Geometry: final body of the model. Coordinates: model frame, mm. A direction names the side the tool comes from. Give positions to 0.01 mm unless a question says otherwise; leave off trailing zeros. Loops run counter-clockwise (first coordinate to the right, second up) from the corner with the lowest first, then second, coordinate; pieces in that order, holes last. Notation, with made-up numbers: (63, 13) -> (119, 13) arc R14 ccw to (119, 32) -> close; hole circle Ø2 at (3.25, 59.25). An arc over 180 degrees is marked (long way). Answer in a Markdown table with one row per item. Add a question column.
1) First-contact query: P1, Ø3, axis at x = 21.5, y = 46, coming from the -Z side; P2, Ø10, axis at x = 134.5, z = -18, coming from the +Y side; P3, Ø10, axis at x = 39, y = -173, coming from the +Z side. Flat tips, straight axial feed; report the tip coordinate or a pass-through.
2) Section query A-A (x = -71). Return the cut outline in (y, z).
3) Line query: line 1 (Y direction, x = -7.5, z = 64); line 2 (X direction, y = -11.5, z = 64.5); line 3 (Y direction, x = 137, z = 19). Output: solid intervals per line, ascending. Write a range as from..to.
4) Draft query along Y for faces 1 (the flat face through (38, -292.151, 36)), 2 (the flat face through (39, -157.151, 35)), 3 (the flat face through (13, -150, 70)), 4 (the flat face through (31, 202.849, 35)). Return one class per face: +Y half, -Y half, draft (parallel to the pull), parting line (faces both ways), or undercut.
5) Section query D-D (x = -150). Return the cut outline in (y, z), plus the area to 3 significant figures.
6) Access query for faces 5 (the flat face through (0, -216, 13)), 6 (the flat face through (80, -216, 12)), 7 (the flat face through (32, 25, 60)), 8 (the flat face through (31, 20, 0)). Directions: +Z, -Z, +X, -X, +Y, -Y. A direction counts if a zero-diameter tool reaches every point of the face in a straight line with its end or side. Return the directions, or none.
7) Section query B-B (y = 135). Return the cut outline in (x, z), plus the area to 3 significant figures.
8) Section query C-C (z = 82). Return the cut outline in (x, y).
Autodesk Inventor part; units mm, degrees
ref_plane "YZ Plane" through (0, 0, 0) normal (1, 0, 0) x (0, 1, 0)
ref_plane "XZ Plane" through (0, 0, 0) normal (0, 1, 0) x (-1, 0, 0)
ref_plane "XY Plane" through (0, 0, 0) normal (0, 0, 1) x (1, 0, 0)
sketch "Esquisse1" plane through (0, 0, 0) normal (0, 0, 1) x (1, 0, 0)
  line L0 (-242.3239, 202.8486) -> (312.6761, 202.8486)
  line L1 (312.6761, 202.8486) -> (312.6761, -157.1514)
  line L2 (312.6761, -157.1514) -> (-242.3239, -157.1514)
  line L3 (-242.3239, -157.1514) -> (-242.3239, 202.8486)
  point P0 (0, 0)
  dimension "d0" = 555
  dimension "d1" = 360
extrude "Extrusion1" add sketch "Esquisse1" along normal blind 70
fillet "Congé1" radius 10 4 edges at (-242.3239, 202.8486, 35) (-242.3239, -157.1514, 35) (312.6761, -157.1514, 35) (312.6761, 202.8486, 35)
sketch "Esquisse2" plane through (0, 0, 70) normal (0, 0, 1) x (1, 0, 0)
  line L0 (-227.3239, 187.8486) -> (297.6761, 187.8486)
  line L1 (297.6761, 187.8486) -> (297.6761, -142.1514)
  line L2 (297.6761, -142.1514) -> (-227.3239, -142.1514)
  line L3 (-227.3239, -142.1514) -> (-227.3239, 187.8486)
  line L4 (302.6761, 202.8486) -> (-232.3239, 202.8486)
  line L5 (-232.3239, -157.1514) -> (302.6761, -157.1514)
  line L6 (-242.3239, 192.8486) -> (-242.3239, -147.1514)
  line L7 (312.6761, -147.1514) -> (312.6761, 192.8486)
  point P0 (0, 0)
  dimension "d5" = 15
  dimension "d6" = 15
  dimension "d7" = 15
  dimension "d8" = 15
extrude "Extrusion2" cut sketch "Esquisse2" against normal blind 10
sketch "Esquisse3" plane through (-232.3239, -157.1514, 0) normal (0, -1, 0) x (1, 0, 0)
  line L0 (232.3239, 0) -> (312.3239, 0)
  line L1 (312.3239, 0) -> (312.3239, 25)
  line L2 (312.3239, 25) -> (232.3239, 25)
  line L3 (232.3239, 25) -> (232.3239, 0)
  dimension "d11" = 80
  dimension "d12" = 25
extrude "Extrusion3" add sketch "Esquisse3" along normal blind 120
sketch "Esquisse4" plane through (-232.3239, -277.1514, 0) normal (0, -1, 0) x (1, 0, 0)
  line L0 (132.3239, 120) -> (412.3239, 120)
  line L1 (412.3239, 120) -> (412.3239, -50)
  line L2 (412.3239, -50) -> (132.3239, -50)
  line L3 (132.3239, -50) -> (132.3239, 120)
  line L4 (232.3239, 25) -> (232.3239, 0)
  dimension "d15" = 170
  dimension "d16" = 280
  dimension "d17" = 50
  dimension "d18" = 100
extrude "Extrusion4" add sketch "Esquisse4" along normal blind 15
fillet "Congé2" radius 10 4 edges at (180, -284.6514, 120) (-100, -284.6514, 120) (180, -284.6514, -50) (-100, -284.6514, -50)
fillet "Congé3" radius 5 8 edges at (177.0711, -277.1514, 117.0711) (180, -277.1514, 35) (177.0711, -277.1514, -47.0711) (40, -277.1514, -50) (-97.0711, -277.1514, -47.0711) (-100, -277.1514, 35) (-97.0711, -277.1514, 117.0711) (40, -277.1514, 120)
equation "\"d6\" = d5"
equation "\"d7\" = d5"
equation "\"d8\" = d5"
properties part number "Ecran"
Evaluation:
| question | item | result |
|---|---|---|
| 1 | P1 | z = 0 |
| 1 | P2 | y = -277.15 |
| 1 | P3 | z = 25 |
| 2 | outline | (-292.15, -50) -> (-282.15, -50) arc R5 ccw to (-277.15, -45) -> (-277.15, 115) arc R5 ccw to (-282.15, 120) -> (-292.15, 120) -> close; (-157.15, 0) -> (202.85, 0) -> (202.85, 70) -> (187.85, 70) -> (187.85, 60) -> (-142.15, 60) -> (-142.15, 70) -> (-157.15, 70) -> close |
| 3 | line 1 | -292.15..-277.15, -157.15..-142.15, 187.85..202.85 |
| 3 | line 2 | -242.32..-227.32, 297.68..312.68 |
| 3 | line 3 | -292.15..-277.15, -157.15..202.85 |
| 4 | face 1 | -Y half |
| 4 | face 2 | undercut |
| 4 | face 3 | draft |
| 4 | face 4 | +Y half |
| 5 | outline | (-157.15, 0) -> (202.85, 0) -> (202.85, 70) -> (187.85, 70) -> (187.85, 60) -> (-142.15, 60) -> (-142.15, 70) -> (-157.15, 70) -> close |
| 5 | area | 21,900 mm² |
| 6 | face 5 | +Z, -Z, -X |
| 6 | face 6 | +Z, -Z, +X |
| 6 | face 7 | +Z |
| 6 | face 8 | -Z, +X, -X, +Y |
| 7 | outline | (-242.32, 0) -> (312.68, 0) -> (312.68, 70) -> (297.68, 70) -> (297.68, 60) -> (-227.32, 60) -> (-227.32, 70) -> (-242.32, 70) -> close |
| 7 | area | 33,600 mm² |
| 8 | outline | (-100, -292.15) -> (180, -292.15) -> (180, -282.15) arc R5 ccw to (175, -277.15) -> (-95, -277.15) arc R5 ccw to (-100, -282.15) -> close |
